Design review of the part built by this model. Coordinates are the model's own, in mm. Coordinates: 2 decimals unless noted, no trailing zeros. Loops run counter-clockwise (first coordinate to the right, second up) from the corner with the lowest first, then second, coordinate; pieces in that order, holes last. Notation, with made-up numbers: (55, 51.25) - (59, 51.25) arc R29 cw to (59, 83.25) - close; hole circle Ø8 at (46.25, -39). An arc over 180 degrees is marked (long way). One line per question, with ' | ' between items.
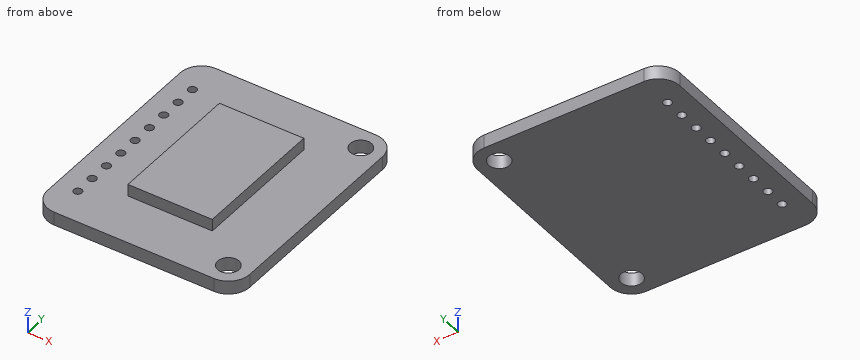
from build123d import *

# Parameters (mm, degrees)
SKETCH1_W           = 24.15
SKETCH1_H           = 28.25
BOSS_EXTRUDE1_DEPTH = 1.6
SKETCH2_R           = 1.27
CUT_EXTRUDE1_DEPTH  = 19.651575001
FILLET1_R           = 2.54
SKETCH3_R           = 0.5
CUT_EXTRUDE2_DEPTH  = 19.651575001
LPATTERN1_COUNT     = 5
LPATTERN1_PITCH     = 2.5
LPATTERN1_COL_COUNT = 5
LPATTERN1_COL_PITCH = 2.5
SKETCH4_W           = 10.07376305
SKETCH4_H           = 15.97396984
BOSS_EXTRUDE2_DEPTH = 1.43


with BuildPart() as part:
    # Sketch1 → Boss-Extrude1 (new body)
    with BuildSketch(Plane.XY):
        Rectangle(SKETCH1_W, SKETCH1_H)
    extrude(amount=BOSS_EXTRUDE1_DEPTH)

    # Sketch2 → Cut-Extrude1 (cut, through all)
    with BuildSketch(Plane.XY.offset(1.6)):
        with Locations((9.505, 11.557)):
            Circle(SKETCH2_R)
        with Locations((9.505, -11.557)):
            Circle(SKETCH2_R)
    extrude(amount=-CUT_EXTRUDE1_DEPTH, mode=Mode.SUBTRACT)

    # Fillet1
    fillet1_edges = [part.edges().sort_by_distance(p)[0] for p in [
        (12.075, -14.125, 0.8),
        (-12.075, -14.125, 0.8),
        (-12.075, 14.125, 0.8),
        (12.075, 14.125, 0.8),
    ]]
    fillet(fillet1_edges, radius=FILLET1_R)

    # Sketch3 → Cut-Extrude2 (cut, through all)
    with BuildSketch(Plane.XY.offset(1.6)):
        with Locations((-9.535, 0)):
            Circle(SKETCH3_R)
    cut_extrude2 = extrude(amount=-CUT_EXTRUDE2_DEPTH, mode=Mode.SUBTRACT)

    # LPattern1: Cut-Extrude2 ×5
    with Locations(*[(0, -i * LPATTERN1_PITCH, 0) for i in range(1, LPATTERN1_COUNT)]):
        add(cut_extrude2, mode=Mode.SUBTRACT)

    # LPattern1 col: Cut-Extrude2 ×5
    with Locations(*[(0, i * LPATTERN1_COL_PITCH, 0) for i in range(1, LPATTERN1_COL_COUNT)]):
        add(cut_extrude2, mode=Mode.SUBTRACT)

    # Sketch4 → Boss-Extrude2 (add)
    with BuildSketch(Plane.XY.offset(1.6)):
        with Locations((0.008744266, 0.138172191)):
            Rectangle(SKETCH4_W, SKETCH4_H)
    extrude(amount=BOSS_EXTRUDE2_DEPTH)


solid = part.part
Q1. Take a section at C-C (z = 0.35). State how many separate pieces and enclosed holes the cut face has, plus the area to 3 significant figures.
Returned:
separate pieces: 1 | enclosed holes: 11 | area: 659 mm²
Q2. Take a section at B-B (x = 1.25). Give the boundary of the cut face in (y, z) (3 decimals), plus the area to 3 significant figures.
Returned:
outline: (-14.125, 0) - (14.125, 0) - (14.125, 1.6) - (8.125, 1.6) - (8.125, 3.03) - (-7.849, 3.03) - (-7.849, 1.6) - (-14.125, 1.6) - close | area: 68.0 mm²
Q3. Take a section at D-D (z = 1.9). Give the boundary of the cut face in (x, y), plus the area to 3 significant figures.
Returned:
outline: (-5.03, -7.85) - (5.05, -7.85) - (5.05, 8.13) - (-5.03, 8.13) - close | area: 161 mm²
Q4. For pin 1 (2 mm diameter, centred on x = 9.505, y = 11.557, fed in from +Z); pin 2 (0.7 mm diameter, centred on x = 2.5, z = 2.5, fed in from +Y); pin 3 (0.7 mm diameter, centred on y = -2.5, z = 2, fed in from +X); pin 4 (1.6 mm diameter, centred on y = 3, z = 2.5, fed in from -X), all flat-tipped, find the tip position at first contact; note any pin that passes through.
Returned:
pin 1: passes through | pin 2: stops at y = 8.13 | pin 3: stops at x = 5.05 | pin 4: stops at x = -5.03
Q5. Take a section at A-A (y = 5). Give the boundary of the cut face in (x, z) (3 decimals), plus the area to 3 significant figures.
Returned:
outline: (-12.075, 0) - (-10.035, 0) - (-10.035, 1.6) - (-12.075, 1.6) - close; (-9.035, 0) - (12.075, 0) - (12.075, 1.6) - (5.046, 1.6) - (5.046, 3.03) - (-5.028, 3.03) - (-5.028, 1.6) - (-9.035, 1.6) - close | area: 51.4 mm²
Q6. To check wall thickness, follow line 1 along Y through (x, z) = (10.25, 0.85); line 2 along Y through (x, z) = (8.75, 0.3) (3 decimals); line 3 along Y through (x, z) = (-3, 2.95). State the ranges of each line that lie inside material, in increasing order.
Returned:
line 1: y = -14.02 to -12.59, -10.53 to 10.53, 12.59 to 14.02 | line 2: y = -14.125 to -12.578, -10.536 to 10.536, 12.578 to 14.125 | line 3: y = -7.85 to 8.13
